Part print with two shaded views. Sizes in mm from the minimum x, y, z corner. A direction names the side the tool comes from. Give positions to 0.01 mm unless a question says otherwise; leave off trailing zeros. Write each loop counter-clockwise with the first axis right and the second up, starting at its lowest first coordinate (ties: lowest second). Pieces come first, ordered by that corner, then holes.
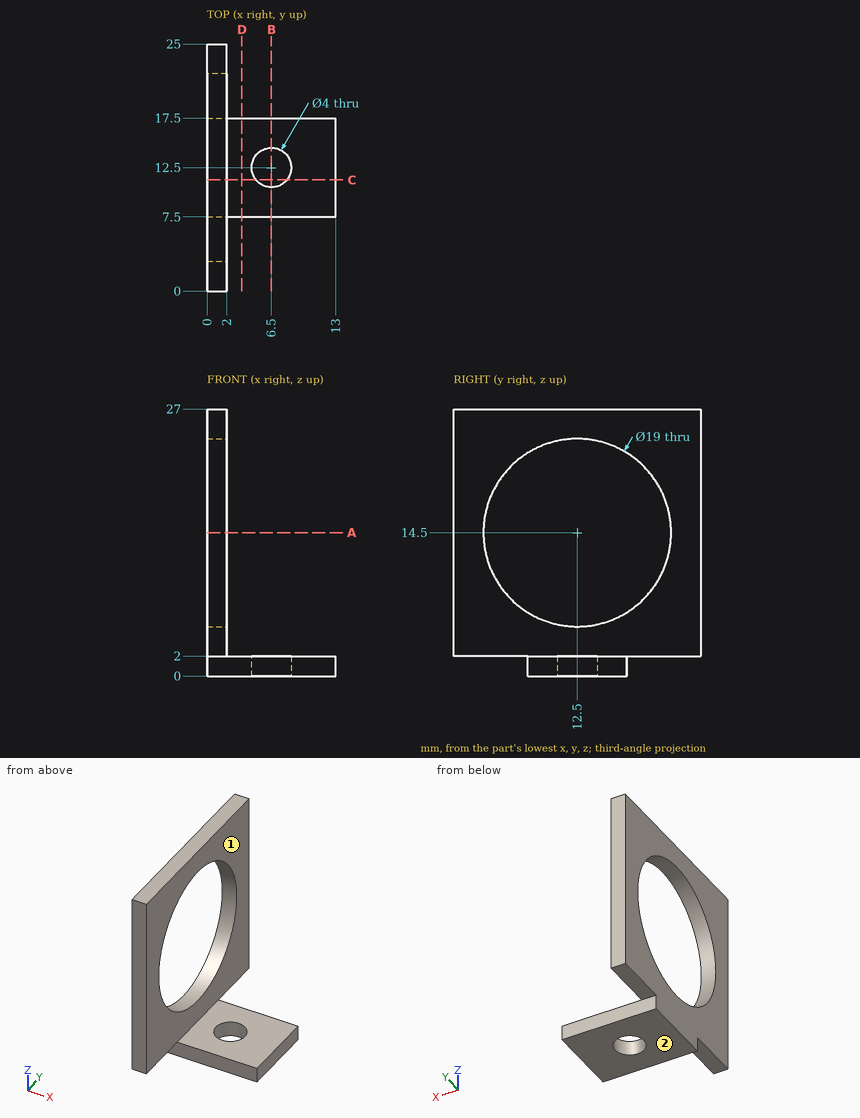
1) Saw through at B-B, the plane x = 6.5. Write the cut outline in (y, z).
Answers follow:
outline: (7.5, 0) - (10.5, 0) - (10.5, 2) - (7.5, 2) - close; (14.5, 0) - (17.5, 0) - (17.5, 2) - (14.5, 2) - close
2) Saw through at A-A, the plane z = 14.5. Write the cut outline in (x, y).
Answers follow:
outline: (0, 0) - (2, 0) - (2, 3) - (0, 3) - close; (0, 22) - (2, 22) - (2, 25) - (0, 25) - close
3) Saw through at C-C, the plane y = 11.25. Write the cut outline in (x, z).
Answers follow:
outline: (0, 0) - (4.94, 0) - (4.94, 2) - (2, 2) - (2, 5.08) - (0, 5.08) - close; (0, 23.92) - (2, 23.92) - (2, 27) - (0, 27) - close; (8.06, 0) - (13, 0) - (13, 2) - (8.06, 2) - close
4) Saw through at D-D, the plane x = 3.5. Write the cut outline in (y, z), then the cut area to 3 significant figures.
Answers follow:
outline: (7.5, 0) - (17.5, 0) - (17.5, 2) - (7.5, 2) - close
area: 20.0 mm2
5) Wall check: L1, parallel to Z at x = 1.3, y = 12.5; L2, parallel to Y at x = 6.5, z = 1.35; L3, parallel to Z at x = 11, y = 12.25. Give the ranges that are in metal, low to high.
Answers follow:
L1: z = 0 to 5, 24 to 27
L2: y = 7.5 to 10.5, 14.5 to 17.5
L3: z = 0 to 2
6) 3-axis set-ups, long thin cutter, end or side, ignore diameter. For the marked faces 1 and 2: which of +Z, -Z, +X, -X, +Y, -Y reach the whole face in a straight line?
Answers follow:
face 1: +Z, +X, +Y, -Y
face 2: -Z, +X, -X, +Y, -Y
7) Pin check, flat tips, straight feed: pin 1 Ø1.6 at (x, y) = (1, 23) entering from -Z; pin 2 Ø3.5 at (x, y) = (6.5, 12.5) entering from +Z; pin 3 Ø1 at (x, z) = (3.5, 1) entering from -Y; pin 4 Ø2 at (x, z) = (6.5, 1) entering from +Y. Stop position of each tip, or through.
Answers follow:
pin 1: stops at z = 2
pin 2: passes through
pin 3: stops at y = 7.5
pin 4: stops at y = 17.5
